The drawing under review shows one solid part. Ordinate dimensions are in mm from its lowest x, y, z. Coordinates: 2 decimals unless noted, no trailing zeros. Order: outer loops, then holes, each group sorted by start corner. A loop starts at its lowest first (then second) coordinate and runs counter-clockwise, first axis right, second up.
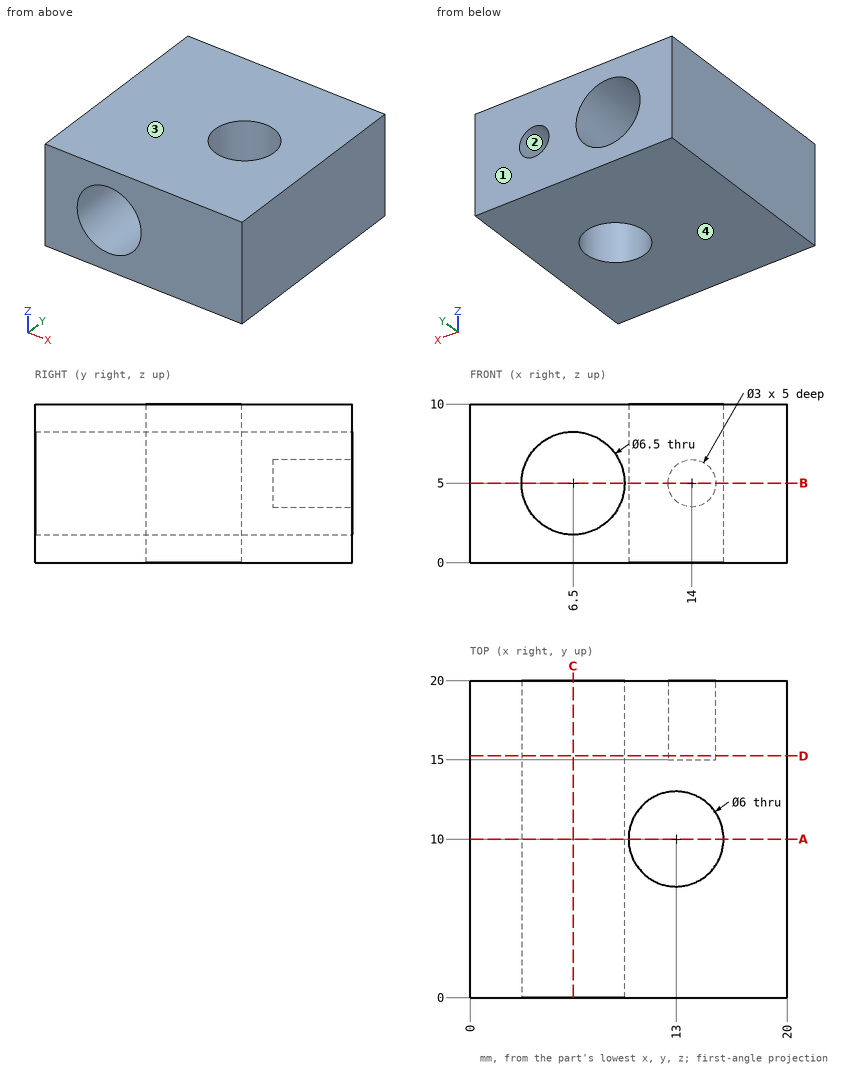
(1) Wall thickness on probe 1 along Y at (x, z) = (13, 5.5); probe 2 along Z at (x, y) = (14, 18.4); probe 3 along Y at (x, z) = (13, 7): over which ranges is each line inside the solid? List them lowest first.
A:
probe 1: y = 0 to 7, 13 to 15
probe 2: z = 0 to 3.5, 6.5 to 10
probe 3: y = 0 to 7, 13 to 20
(2) We need section C-C, the plane x = 6.5. Write out the cut boundary in (y, z), and give its area (3 significant figures).
A:
outline: (0, 0) - (20, 0) - (20, 1.75) - (0, 1.75) - close; (0, 8.25) - (20, 8.25) - (20, 10) - (0, 10) - close
area: 70.0 mm2
(3) We need section D-D, the plane y = 15.25. Write out the cut boundary in (x, z).
A:
outline: (0, 0) - (20, 0) - (20, 10) - (0, 10) - close; hole circle Ø6.5 at (6.5, 5); hole circle Ø3 at (14, 5)
(4) We need section A-A, the plane y = 10. Write out the cut boundary in (x, z), and give its area (3 significant figures).
A:
outline: (0, 0) - (10, 0) - (10, 10) - (0, 10) - close; (16, 0) - (20, 0) - (20, 10) - (16, 10) - close; hole circle Ø6.5 at (6.5, 5)
area: 107 mm2
(5) For pin 1 Ø1.5 at (y, z) = (11, 5.5) entering from -X, flat-tipped, find the tip position at first contact; note if it passes through.
A:
pin 1: stops at x = 0
(6) We need section B-B, the plane z = 5. Write out the cut boundary in (x, y).
A:
outline: (0, 0) - (3.25, 0) - (3.25, 20) - (0, 20) - close; (9.75, 0) - (20, 0) - (20, 20) - (15.5, 20) - (15.5, 15) - (12.5, 15) - (12.5, 20) - (9.75, 20) - close; hole circle Ø6 at (13, 10)
(7) Draft analysis for pull direction Z (two halves, no side actions). For the marked faces 1, 2, 3 and 4, state which applies: released by +Z, released by -Z, zero draft, split by the parting line, or undercut.
A:
face 1: zero draft
face 2: undercut
face 3: released by +Z
face 4: released by -Z
